Check sheet for the modelled part. Datum: model origin and axes. Units: mm. A direction names the side the tool comes from. Give positions to 0.01 mm unless a question says otherwise; leave off trailing zeros. Loops run counter-clockwise (first coordinate to the right, second up) from the corner with the lowest first, then second, coordinate; pieces in that order, holes last. Notation, with made-up numbers: M 79.25,-22.5 L 119.25,-22.5 A16 cw 119.25,-0.5 Z; hole C 65,78 d1. An arc over 180 degrees is marked long. Write each question's results on one line, items separated by ' | '. Start each with the question number.
1. Sectioned sample at A-A on y = 21.5. Record the cut outline in (x, z).
2. Sectioned sample at C-C on y = -16.5. Record the cut outline in (x, z) (3 decimals).
3. Sectioned sample at D-D on z = 0.2. Give the number of separate pieces and of enclosed holes in the cut face, and give its area (3 significant figures).
4. Tool access check on faces 1 (the flat face through (-5.166, -12.626, 0.592)), 2 (the flat face through (-12.1, -23.9, 0.6)), 3 (the flat face through (0.87, 24.66, 0.59)). Record the directions out of +Z, -Z, +X, -X, +Y, -Y that give a thin tool (end or side, any length) a straight path to the whole face; none if there is none.
5. Draft check along Y on faces 4 (the flat face through (-6, 10, 0)), 5 (the flat face through (21.77, -11.59, 0.59)), 6 (the flat face through (2.5, 16, 1)). Enter one of: pulls with the +Y half, pulls with the -Y half, needs draft (parallel to the pull), parting line crosses it, or undercut.
6. Sectioned sample at B-B on x = -8.5. Record the cut outline in (y, z), and give its area (3 significant figures).
7. Go/stop test with flat-tipped pins: pin 1 (0.6 mm diameter, centred on y = 16, z = 0.5, fed in from -X); pin 2 (0.6 mm diameter, centred on y = -12.5, z = 0.5, fed in from +X); pin 3 (0.6 mm diameter, centred on x = -8, z = 0.5, fed in from -Y). Record where each tip stops, or that it passes through.
8. Material ranges on line 1 along Y through (x, z) = (7, 0.75); line 2 along X through (y, z) = (-9, 0.3); line 3 along X through (y, z) = (10.5, 0.2), recorded low to high.
```python
from build123d import *

# Parameters (mm, degrees)
BASE_DEPTH               = 1.2
PCB_SKETCH_W             = 4.450002
PCB_SKETCH_H             = 7.250001
PCB_COMPONENT_ROOM_DEPTH = 40.187510032
REMOVAL_ROOM_SIZE        = 1


with BuildPart() as part:
    # Base sketch → Base (new body)
    with BuildSketch(Plane.XY):
        with BuildLine():
            Line((22.639032554, -11.088045382), (26.75, -3.967640898))
            Line((26.75, -3.967640898), (26.75, 7.167640898))
            add(Edge.make_bspline(
                [(19.582359102, 19.582359102), (26.75, 15.444119701), (26.75, 7.167640898)],
                knots=[0, 0, 0, 1, 1, 1], degree=2, weights=[1, 0.818181818, 1]))
            Line((19.582359102, 19.582359102), (9.93892219, 25.15))
            Line((9.93892219, 25.15), (1.716987298, 25.15))
            Line((1.716987298, 25.15), (0, 24.158696921))
            Line((0, 24.158696921), (-1.716987298, 25.15))
            Line((-1.716987298, 25.15), (-9.93892219, 25.15))
            Line((-9.93892219, 25.15), (-19.582359102, 19.582359102))
            add(Edge.make_bspline(
                [(-19.582359102, 19.582359102), (-26.75, 15.444119701), (-26.75, 7.167640898)],
                knots=[0, 0, 0, 1, 1, 1], degree=2, weights=[1, 0.818181818, 1]))
            Line((-26.75, 7.167640898), (-26.75, -3.967640898))
            Line((-26.75, -3.967640898), (-22.639032554, -11.088045382))
            Line((-22.639032554, -11.088045382), (-20.922045256, -12.079348461))
            Line((-20.922045256, -12.079348461), (-20.922045256, -14.061954618))
            Line((-20.922045256, -14.061954618), (-16.81107781, -21.182359102))
            Line((-16.81107781, -21.182359102), (-7.167640898, -26.75))
            add(Edge.make_bspline(
                [(7.167640898, -26.75), (0, -30.888239402), (-7.167640898, -26.75)],
                knots=[0, 0, 0, 1, 1, 1], degree=2, weights=[1, 0.818181818, 1]))
            Line((7.167640898, -26.75), (16.81107781, -21.182359102))
            Line((16.81107781, -21.182359102), (20.922045256, -14.061954618))
            Line((20.922045256, -14.061954618), (20.922045256, -12.079348461))
            Line((20.922045256, -12.079348461), (22.639032554, -11.088045382))
        make_face()
    extrude(amount=BASE_DEPTH)

    # PCB sketch → PCB Component room (cut, through all)
    # profile 1 of 7: a face of its own
    with BuildSketch(Plane.XY):
        with Locations((-8.341529649, 14.3760387)):
            Rectangle(PCB_SKETCH_W, PCB_SKETCH_H)
    # profile 2 of 7: a face of its own
    with BuildSketch(Plane.XY):
        with BuildLine():
            Line((7.292235248, -7.096920387), (17.939993848, -13.244411362))
            Line((17.939993848, -13.244411362), (22.271882405, -5.741366))
            ThreePointArc((22.271882405, -5.741366), (22.817247788, -2.893669145), (23.000004364, 1.377e-05))
            ThreePointArc((23.000004364, 1.377e-05), (21.859361277, 7.153230156), (18.550568269, 13.596944935))
            Line((18.550568269, 13.596944935), (7.292237734, 7.096945429))
            Line((7.292237734, 7.096945429), (2.500009052, 9.863735785))
            Line((2.500009052, 9.863735785), (2.500009052, 22.158696921))
            Line((2.500009052, 22.158696921), (-2.499990948, 22.158696921))
            Line((-2.499990948, 22.158696921), (-2.499990948, 9.863735785))
            Line((-2.499990948, 9.863735785), (-7.292227753, 7.096933454))
            Line((-7.292227753, 7.096933454), (-18.550555859, 13.596937166))
            ThreePointArc((-18.550555859, 13.596937166), (-19.91857187, 11.500010223), (-21.050555597, 9.266809996))
            Line((-21.050555597, 9.266809996), (-9.792227491, 2.766806284))
            Line((-9.792227491, 2.766806284), (-9.792228638, -2.766774829))
            Line((-9.792228638, -2.766774829), (-20.440003139, -8.91426968))
            Line((-20.440003139, -8.91426968), (-17.940003329, -13.244396808))
            Line((-17.940003329, -13.244396808), (-7.29223057, -7.096902963))
            Line((-7.29223057, -7.096902963), (-2.499990948, -9.863708244))
            Line((-2.499990948, -9.863708244), (-2.499990948, -22.863708244))
            ThreePointArc((-2.499990948, -22.863708244), (9.052e-06, -22.999981541), (2.500009052, -22.863708244))
            Line((2.500009052, -22.863708244), (2.500009052, -9.863708244))
            Line((2.500009052, -9.863708244), (7.292235248, -7.096920387))
        make_face()
        Polygon((14.573158226, 3.739426369), (20.85184327, 0.114425869), (18.62684227, -3.73938891), (12.348157226, -0.11438841), align=None, mode=Mode.SUBTRACT)
    # profile 3 of 7: a face of its own
    with BuildSketch(Plane.XY):
        Polygon((20.85184327, 0.114425869), (14.573158226, 3.739426369), (12.348157226, -0.11438841), (18.62684227, -3.73938891), align=None)
    # profile 4 of 7: a face of its own
    with BuildSketch(Plane.XY):
        with Locations((8.300001248, -14.39998027)):
            Rectangle(PCB_SKETCH_W, PCB_SKETCH_H)
    # profile 5 of 7: a face of its own
    with BuildSketch(Plane.XY):
        Polygon((-10.347605222, -18.151377424), (-4.068920179, -14.526376924), (-6.293921179, -10.672562146), (-12.572606222, -14.297562646), align=None)
    # profile 6 of 7: a face of its own
    with BuildSketch(Plane.XY):
        Polygon((10.306076821, 18.127435854), (4.027391778, 14.502435354), (6.252392778, 10.648620576), (12.531077821, 14.273621076), align=None)
    # profile 7 of 7: a face of its own
    with BuildSketch(Plane.XY):
        Polygon((-20.893371671, -0.138367439), (-14.614686627, -3.763367939), (-12.389685627, 0.09044684), (-18.668370671, 3.71544734), align=None)
    extrude(amount=PCB_COMPONENT_ROOM_DEPTH, mode=Mode.SUBTRACT)

    # Removal room
    removal_room_edges = [part.edges().sort_by_distance(p)[0] for p in [
        (22.585630976, 4.346215175, 0),
    ]]
    chamfer(removal_room_edges, length=REMOVAL_ROOM_SIZE)


solid = part.part
```
Output values:
1) outline: M -16.26,0 L -2.5,0 L -2.5,1.2 L -16.26,1.2 Z; M 2.5,0 L 16.26,0 L 16.26,1.2 L 2.5,1.2 Z
2) outline: M -19.514,0 L -11.301,0 L -11.301,1.2 L -19.514,1.2 Z; M -7.487,0 L -2.5,0 L -2.5,1.2 L -7.487,1.2 Z; M 2.5,0 L 6.075,0 L 6.075,1.2 L 2.5,1.2 Z; M 10.525,0 L 19.514,0 L 19.514,1.2 L 10.525,1.2 Z
3) separate pieces: 1 | enclosed holes: 6 | area: 1,240 mm2
4) face 1: +Z, -Z | face 2: +Z, -Z, -X, -Y | face 3: +Z, -Z, +Y
5) face 4: needs draft | face 5: pulls with the -Y half | face 6: undercut
6) outline: M -25.98,0 L -17.08,0 L -17.08,1.2 L -25.98,1.2 Z; M -11.95,0 L -7.79,0 L -7.79,1.2 L -11.95,1.2 Z; M 7.79,0 L 10.75,0 L 10.75,1.2 L 7.79,1.2 Z; M 18,0 L 25.15,0 L 25.15,1.2 L 18,1.2 Z | area: 27.8 mm2
7) pin 1: x = -23.87 | pin 2: x = 20.92 | pin 3: y = -26.44
8) line 1: -26.85 to -18.02, -10.77 to -7.27, 7.27 to 11.08, 16.22 to 25.15 | line 2: -23.84 to -20.39, -10.59 to -4, 4 to 10.59, 20.39 to 23.84 | line 3: -26.33 to -20.46, -13.19 to -2.5, 2.5 to 13.19, 21.36 to 26.33
